The listing builds one solid part. Answer for the finished solid, in the listing's coordinates (mm). Face numbers are marked on the shaded views. A direction names the side the tool comes from. Round coordinates to 2 decimals unless told otherwise and drop trailing zeros. Write each loop counter-clockwise with the first axis right and the second up, starting at its lowest first coordinate (ties: lowest second). Pieces come first, ordered by that corner, then holes. Notation, with made-up numbers: (64.25, 67.25) - (103.25, 67.25) arc R35 cw to (103.25, 104.25) - close; hole circle Ø10 at (48, -37.75). An arc over 180 degrees is marked (long way). Answer in a Markdown table with one row per item.
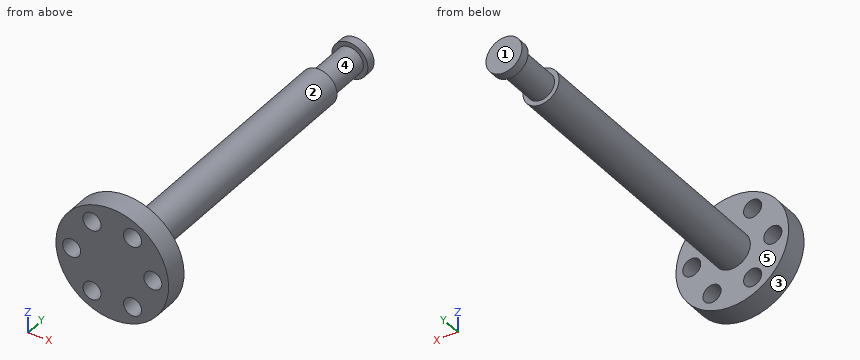
from build123d import *

# Parameters (mm, degrees)
SKETCH_1_R               = 12.5
EXTRUDE_1_DEPTH          = 79
SKETCH_2_OUTSIDE_W       = 44.31
SKETCH_2_OUTSIDE_H       = 44.31
SKETCH_2_OUTSIDE_R       = 4
CUT_EXTRUDE_2_DEPTH      = 72
SKETCH_4_OUTSIDE_W       = 44.31
SKETCH_4_OUTSIDE_H       = 44.31
SKETCH_4_OUTSIDE_R       = 4
CUT_EXTRUDE_3_DEPTH      = 80.003164494
SKETCH_6_OUTSIDE_W       = 44.31
SKETCH_6_OUTSIDE_H       = 44.31
SKETCH_6_OUTSIDE_R       = 3
CUT_EXTRUDE_4_DEPTH      = 10
SKETCH_7_R               = 2
CUT_EXTRUDE_5_DEPTH      = 81.953690466
PATTERN_CIRCULAR_1_COUNT = 6


with BuildPart() as part:
    # 草图1 → 凸台-拉伸1 (new body)
    with BuildSketch(Plane(origin=(0, 0, 0), x_dir=(1, 0, 0), z_dir=(0, 1, 0))):
        with Locations(Location((0, 0, 0), (0, 0, 270))):
            Circle(SKETCH_1_R)
    extrude(amount=EXTRUDE_1_DEPTH)

    # 草图2 outside → 切除-拉伸2 (cut)
    with BuildSketch(Plane(origin=(0, 77, 0), x_dir=(1, 0, 0), z_dir=(0, 1, 0))):
        Rectangle(SKETCH_2_OUTSIDE_W, SKETCH_2_OUTSIDE_H)
        with Locations(Location((0, 0, 0), (0, 0, 270))):
            Circle(SKETCH_2_OUTSIDE_R, mode=Mode.SUBTRACT)
    extrude(amount=-CUT_EXTRUDE_2_DEPTH, mode=Mode.SUBTRACT)

    # 草图4 outside → 切除-拉伸3 (cut, through all)
    with BuildSketch(Plane(origin=(0, 77, 0), x_dir=(1, 0, 0), z_dir=(0, 1, 0))):
        Rectangle(SKETCH_4_OUTSIDE_W, SKETCH_4_OUTSIDE_H)
        with Locations(Location((0, 0, 0), (0, 0, 270))):
            Circle(SKETCH_4_OUTSIDE_R, mode=Mode.SUBTRACT)
    extrude(amount=CUT_EXTRUDE_3_DEPTH, mode=Mode.SUBTRACT)

    # 草图6 outside → 切除-拉伸4 (cut)
    with BuildSketch(Plane(origin=(0, 77, 0), x_dir=(1, 0, 0), z_dir=(0, 1, 0))):
        Rectangle(SKETCH_6_OUTSIDE_W, SKETCH_6_OUTSIDE_H)
        with Locations(Location((0, 0, 0), (0, 0, 270))):
            Circle(SKETCH_6_OUTSIDE_R, mode=Mode.SUBTRACT)
    extrude(amount=-CUT_EXTRUDE_4_DEPTH, mode=Mode.SUBTRACT)

    # 草图7 → 切除-拉伸5 (cut, through all)
    with BuildSketch(Plane.XZ):
        with Locations(Location((9, 0, 0), (0, 0, 270))):
            Circle(SKETCH_7_R)
    cut_extrude_5 = extrude(amount=-CUT_EXTRUDE_5_DEPTH, mode=Mode.SUBTRACT)

    # 阵列(圆周)1: 切除-拉伸5 ×6 about axis
    pattern_circular_1_axis = Axis((0, 0, 0), (0, 1, 0))
    for i in range(1, PATTERN_CIRCULAR_1_COUNT):
        add(cut_extrude_5.rotate(pattern_circular_1_axis, i * 360 / PATTERN_CIRCULAR_1_COUNT), mode=Mode.SUBTRACT)


solid = part.part
(1) For the marked faces 1 and 2, determine the directions among +Z, -Z, +X, -X, +Y, -Y from which every point of the face is accessible in a straight line to the end or side of a thin tool.
Checked values:
| item | result |
|---|---|
| face 1 | +Z, -Z, +X, -X, +Y |
| face 2 | +Y |
(2) Section D-D (z = 8) is taken. Give the vertices of the cut face in (x, y), and give its area (3 significant figures).
Checked values:
| item | result |
|---|---|
| outline | (-9.6, 0) - (-6.49, 0) - (-6.49, 5) - (-9.6, 5) - close; (-2.51, 0) - (2.51, 0) - (2.51, 5) - (-2.51, 5) - close; (6.49, 0) - (9.6, 0) - (9.6, 5) - (6.49, 5) - close |
| area | 56.3 mm2 |
(3) Section C-C (x = 0) is taken. Give the vertices of the cut face in (y, z), and give its area (3 significant figures).
Checked values:
| item | result |
|---|---|
| outline | (0, -12.5) - (5, -12.5) - (5, -4) - (67, -4) - (67, -3) - (77, -3) - (77, -4) - (79, -4) - (79, 4) - (77, 4) - (77, 3) - (67, 3) - (67, 4) - (5, 4) - (5, 12.5) - (0, 12.5) - close |
| area | 697 mm2 |
(4) Section A-A (z = 0) is taken. Give the vertices of the cut face in (x, y), and give its area (3 significant figures).
Checked values:
| item | result |
|---|---|
| outline | (-12.5, 0) - (-11, 0) - (-11, 5) - (-12.5, 5) - close; (-7, 0) - (7, 0) - (7, 5) - (4, 5) - (4, 67) - (3, 67) - (3, 77) - (4, 77) - (4, 79) - (-4, 79) - (-4, 77) - (-3, 77) - (-3, 67) - (-4, 67) - (-4, 5) - (-7, 5) - close; (11, 0) - (12.5, 0) - (12.5, 5) - (11, 5) - close |
| area | 657 mm2 |
(5) For a pull along Y with two mould halves and no side action, classify the marked faces 3, 4 and 5 as pulls with the +Y half, pulls with the -Y half, needs draft (parallel to the pull), parting line crosses it, or undercut.
Checked values:
| item | result |
|---|---|
| face 3 | needs draft |
| face 4 | undercut |
| face 5 | pulls with the +Y half |
(6) Flat-ended cylindrical pins translate along their axes: pin 1 (8 mm diameter, centred on y = 43, z = 2.5, fed in from +X); pin 2 (6.5 mm diameter, centred on x = 4.5, z = -7.79, fed in from +Y); pin 3 (12 mm diameter, centred on y = 48, z = 6.5, fed in from -X). Find the tip coordinate at first contact, or state that the pin passes through.
Checked values:
| item | result |
|---|---|
| pin 1 | stops at x = 4 |
| pin 2 | stops at y = 5 |
| pin 3 | stops at x = -3.97 |
(7) Section B-B (x = -9) is taken. Give the vertices of the cut face in (y, z), and give its area (3 significant figures).
Checked values:
| item | result |
|---|---|
| outline | (0, -8.67) - (5, -8.67) - (5, -2) - (0, -2) - close; (0, 2) - (5, 2) - (5, 8.67) - (0, 8.67) - close |
| area | 66.7 mm2 |
(8) Find the intervals of material crossed by line 1 (X direction, y = 2.9, z = 0); line 2 (X direction, y = 4, z = -1.75); line 3 (Y direction, x = -5.75, z = -3.5), in increasing order.
Checked values:
| item | result |
|---|---|
| line 1 | x = -12.5 to -11, -7 to 7, 11 to 12.5 |
| line 2 | x = -12.38 to -9.97, -8.03 to 8.03, 9.97 to 12.38 |
| line 3 | y = 0 to 5 |
